```python
from build123d import *

# Parameters (mm, degrees)
SKETCH1_R           = 1.35
SKETCH1_R_2         = 2.15
BOSS_EXTRUDE1_DEPTH = 6
SKETCH2_R           = 2.15
CUT_EXTRUDE1_DEPTH  = 4.2


with BuildPart() as part:
    # Sketch1 → Boss-Extrude1 (new body)
    with BuildSketch(Plane.XY):
        with BuildLine():
            Line((-16.436457619, 29), (-11.155935204, 29))
            ThreePointArc((-11.155935204, 29), (-9.748616749, 29.926511277), (-9.214880919, 31.524664725))
            ThreePointArc((-9.214880919, 31.524664725), (0, 40.739545643), (9.214880919, 31.524664725))
            ThreePointArc((9.214880919, 31.524664725), (9.748616749, 29.926511277), (11.155935204, 29))
            Line((11.155935204, 29), (17.063542381, 29))
            Line((17.063542381, 29), (17.063542381, -29))
            Line((17.063542381, -29), (11.155935204, -29))
            ThreePointArc((11.155935204, -29), (9.748616749, -29.926511277), (9.214880919, -31.524664725))
            ThreePointArc((9.214880919, -31.524664725), (0, -40.739545643), (-9.214880919, -31.524664725))
            ThreePointArc((-9.214880919, -31.524664725), (-9.748616749, -29.926511277), (-11.155935204, -29))
            Line((-11.155935204, -29), (-16.436457619, -29))
            Line((-16.436457619, -29), (-16.436457619, 29))
        make_face()
        with Locations((-13.5, 25.3)):
            Circle(SKETCH1_R, mode=Mode.SUBTRACT)
        with Locations((13.5, -25.3)):
            Circle(SKETCH1_R, mode=Mode.SUBTRACT)
        with Locations((-13.5, -25.3)):
            Circle(SKETCH1_R, mode=Mode.SUBTRACT)
        with Locations((13.5, 25.3)):
            Circle(SKETCH1_R, mode=Mode.SUBTRACT)
        with Locations((0, 35)):
            Circle(SKETCH1_R_2, mode=Mode.SUBTRACT)
        with Locations(Location((0, -35, 0), (0, 0, 180))):
            Circle(SKETCH1_R_2, mode=Mode.SUBTRACT)
        with BuildLine():
            Line((-13.5, 16), (13.5, 16))
            Line((13.5, 16), (13.5, -16))
            Line((13.5, -16), (-0.3, -16))
            ThreePointArc((-0.3, -16), (-0.921986523, -15.060993262), (-1.3, -14))
            ThreePointArc((-1.3, -14), (-1.678013477, -15.060993262), (-2.3, -16))
            Line((-2.3, -16), (-13.5, -16))
            Line((-13.5, -16), (-13.5, 16))
        make_face(mode=Mode.SUBTRACT)
    extrude(amount=BOSS_EXTRUDE1_DEPTH)

    # Sketch2 → Cut-Extrude1 (cut)
    with BuildSketch(Plane.XY.offset(6)):
        with Locations((-12, 20)):
            Circle(SKETCH2_R)
        with Locations((-6, 20)):
            Circle(SKETCH2_R)
        with Locations((0, 20)):
            Circle(SKETCH2_R)
        with Locations((6, 20)):
            Circle(SKETCH2_R)
        with Locations((12, 20)):
            Circle(SKETCH2_R)
        with Locations((-6, 26)):
            Circle(SKETCH2_R)
        with Locations((0, 26)):
            Circle(SKETCH2_R)
        with Locations((6, 26)):
            Circle(SKETCH2_R)
        with Locations((-11.967349369, -20)):
            Circle(SKETCH2_R)
        with Locations((-5.983674685, -20)):
            Circle(SKETCH2_R)
        with Locations((0, -20)):
            Circle(SKETCH2_R)
        with Locations((5.983674685, -20)):
            Circle(SKETCH2_R)
        with Locations((11.967349369, -20)):
            Circle(SKETCH2_R)
        with Locations((-5.983674685, -26)):
            Circle(SKETCH2_R)
        with Locations((0, -26)):
            Circle(SKETCH2_R)
        with Locations((5.983674685, -26)):
            Circle(SKETCH2_R)
    extrude(amount=-CUT_EXTRUDE1_DEPTH, mode=Mode.SUBTRACT)


solid = part.part
```
Source: CAD feature listing. Evaluate the final solid. Frame: model axes, mm. A direction names the side the tool comes from. Round coordinates to 2 decimals unless told otherwise and drop trailing zeros. Loops run counter-clockwise (first coordinate to the right, second up) from the corner with the lowest first, then second, coordinate; pieces in that order, holes last.
1. Access query for faces 1 (the flat face through (15, 1, 6)), 2 (the flat face through (7, -16, 3)), 3 (the flat face through (14, 29, 3)), 4 (the cylindrical face through (-12.43, -22.1, 3.93)). Directions: +Z, -Z, +X, -X, +Y, -Y. A direction counts if a zero-diameter tool reaches every point of the face in a straight line with its end or side. Return the directions, or none.
2. Section query D-D on x = 1. Give the number of separate pieces and of enclosed holes in the cut face, and give its area (3 significant figures).
3. Section query C-C on x = -5. Output: boundary loops of the cut face in (y, z).
4. Section query B-B on z = 0.8. Output: boundary loops of the cut face in (x, y).
5. Contact query for flat-ended pins moving along their axis: pin 1 (1 mm diameter, centred on y = 30, z = 5, fed in from -X); pin 2 (1.3 mm diameter, centred on x = -0.5, y = 19, fed in from +Z); pin 3 (4 mm diameter, centred on x = -10, y = -6.5, fed in from +Z). Output: stop coordinate, or through.
6. Ray query, L1, parallel to X at y = -5, z = 5.6; L2, parallel to Y at x = -10.5, z = 3.3; L3, parallel to Y at x = 11, z = 5.2. Return the intervals inside material, ascending.
7. Mould query, pull axis Y, two halves, no side actions, for faces 5 (the flat face through (-16.436, 0, 3)), 6 (the cylindrical face through (-6.45, -22.1, 3.93)), 7 (the cylindrical face through (0.203, -40.737, 2.958)), 8 (the cylindrical face through (-0.203, 40.737, 2.958)). Classes: released by +Y, released by -Y, zero draft, split by the parting line, or undercut.
8. Section query A-A on y = 4.5. Output: boundary loops of the cut face in (x, z), and give its area (3 significant figures).
Answers below:
1. face 1: +Z, +X, -X, +Y, -Y
1. face 2: +Z, -Z
1. face 3: +Z, -Z, +X, +Y
1. face 4: +Z
2. separate pieces: 4
2. enclosed holes: 0
2. area: 187 mm2
3. outline: (-39.27, 0) - (-16, 0) - (-16, 6) - (-18.09, 6) - (-18.09, 1.8) - (-21.91, 1.8) - (-21.91, 6) - (-24.09, 6) - (-24.09, 1.8) - (-27.91, 1.8) - (-27.91, 6) - (-39.27, 6) - close; (16, 0) - (39.27, 0) - (39.27, 6) - (27.9, 6) - (27.9, 1.8) - (24.1, 1.8) - (24.1, 6) - (21.9, 6) - (21.9, 1.8) - (18.1, 1.8) - (18.1, 6) - (16, 6) - close
4. outline: (-16.44, -29) - (-11.16, -29) arc R2.58 cw to (-9.21, -31.52) arc R9.21 ccw to (9.21, -31.52) arc R2.58 cw to (11.16, -29) - (17.06, -29) - (17.06, 29) - (11.16, 29) arc R2.58 cw to (9.21, 31.52) arc R9.21 ccw to (-9.21, 31.52) arc R2.58 cw to (-11.16, 29) - (-16.44, 29) - close; hole circle Ø2.7 at (-13.5, -25.3); hole circle Ø2.7 at (-13.5, 25.3); hole (-13.5, -16) - (-2.3, -16) arc R4.65 ccw to (-1.3, -14) arc R4.65 ccw to (-0.3, -16) - (13.5, -16) - (13.5, 16) - (-13.5, 16) - close; hole circle Ø4.3 at (0, -35); hole circle Ø4.3 at (0, 35); hole circle Ø2.7 at (13.5, -25.3); hole circle Ø2.7 at (13.5, 25.3)
5. pin 1: stops at x = -10.16
5. pin 2: stops at z = 1.8
5. pin 3: passes through
6. L1: x = -16.44 to -13.5, 13.5 to 17.06
6. L2: y = -29.27 to -21.57, -18.43 to -16, 16 to 18.46, 21.54 to 29.27
6. L3: y = -29.04 to -21.92, -18.08 to -16, 16 to 18.1, 21.9 to 29.04
7. face 5: zero draft
7. face 6: undercut
7. face 7: released by -Y
7. face 8: released by +Y
8. outline: (-16.44, 0) - (-13.5, 0) - (-13.5, 6) - (-16.44, 6) - close; (13.5, 0) - (17.06, 0) - (17.06, 6) - (13.5, 6) - close
8. area: 39.0 mm2
